Autodesk Fusion 360 part; units mm, degrees
sketch "Sketch1" plane through (0, 0, 0) normal (0, 0, 1) x (1, 0, 0)
  circle A0 centre (0, 0) radius 7
  line L0 (-2.1, -1.3565) -> (-2.1, 1.3565)
  arc A1 (-2.1, -1.3565) -> (-2.1, 1.3565) centre (0, 0) ccw
  dimension "d1" = 14
  dimension "d8" = 5
  dimension "d9" = 2.1
extrude "Extrude1" add sketch "Sketch1" along normal blind 22 contours A0 | L0 A1 makes body 1
ref_plane "WorkPlane1" through (0, 0, 40.2) normal (0, 0, 1) x (1, 0, 0)
sketch "Sketch2" plane through (0, 0, 40.2) normal (0, 0, 1) x (1, 0, 0)
  circle A0 centre (0, 0) radius 7
  circle A1 centre (3, 0) radius 4
  dimension "d5" = 8
extrude "Extrude2" add sketch "Sketch2" against normal blind 7.3 separate body contours A1 makes body 2
loft "Loft1" add section 1 face at (3.1171, 1.096, 32.9) section 2 face at (1.11, -1.8763, 22) on bodies 1 2 bodies 1 2
extrude "Extrude3" cut sketch "Sketch1" along normal blind 21 contours L0 A1 bodies 1
chamfer "Chamfer1" distance 0.5 angle 45 1 edges at (-0.7293, -1.4465, 40.2) on bodies 1 2
Could you check a few things on this model? Use its own coordinates, in mm. A direction names the side the tool comes from. Coordinates: 2 decimals unless noted, no trailing zeros. Loops run counter-clockwise (first coordinate to the right, second up) from the corner with the lowest first, then second, coordinate; pieces in that order, holes last.
1) Which directions (+Z, -Z, +X, -X, +Y, -Y) give clear straight access to the entire face, cutting with the end or side of a thin tool? Please do faces 1 (the face through (2.5, 0.1, 10.4)), 2 (the face through (6.466, 2.681, 10.846)).
Reported:
face 1: -Z
face 2: +Z, -Z
2) Please list where these lines run through material, in increasing order: line 1 along Y through (x, z) = (0, 14); line 2 along Y through (x, z) = (-1.25, 17); line 3 along X through (y, z) = (-4, 12).
Reported:
line 1: y = -7 to -2.5, 2.5 to 7
line 2: y = -6.89 to -2.17, 2.17 to 6.89
line 3: x = -5.74 to 5.74
3) Will these pins go through, and if not, where does the flat tip stop? pin 1 Ø5 at (x, z) = (4.5, 7.5) entering from +Y; pin 2 Ø2 at (x, z) = (5, 32.5) entering from +Y; pin 3 Ø1 at (x, z) = (3, 29.5) entering from -Y.
Reported:
pin 1: stops at y = 6.71
pin 2: stops at y = 4.02
pin 3: stops at y = -4.99
4) Thinking about a two-plate mould opening in Y: for faces 3 (the face through (3, 0, 40.2)), 4 (the face through (4.846, -3.549, 36.348)), 5 (the face through (0, 0, 21)), which applies, released by +Y, released by -Y, zero draft, split by the parting line, or undercut?
Reported:
face 3: zero draft
face 4: split by the parting line
face 5: undercut
5) Imagine slicing it at A-A (z = 3). List the corners of the cut face in (x, y) for me.
Reported:
outline: circle Ø14 at (0, 0); hole (-2.1, -1.36) arc R2.5 ccw (long way) to (-2.1, 1.36) - close
6) Imagine slicing it at B-B (z = 36). List the corners of the cut face in (x, y) for me.
Reported:
outline: circle Ø8 at (3, 0)
